from build123d import *

# Parameters (mm, degrees)
SKETCH1_W                = 369
SKETCH1_H                = 203
BOSS_EXTRUDE1_DEPTH      = 20
SKETCH2_W                = 129
SKETCH2_H                = 16
BOSS_EXTRUDE2_DEPTH      = 12
SKETCH3_W                = 342
SKETCH3_H                = 171
CUT_EXTRUDE1_DEPTH       = 9
SKETCH4_W                = 100
SKETCH4_H                = 12
BOSS_EXTRUDE3_DEPTH      = 60
CUT_EXTRUDE3_START       = -60
CUT_EXTRUDE3_DEPTH       = 70
BOSS_EXTRUDE5_DEPTH      = 40
EXTRUDE_THIN1_DEPTH      = 7
SKETCH10_W               = 404
SKETCH10_H               = 324.796202869
CUT_EXTRUDE4_DEPTH       = 69
CUT_EXTRUDE7_DEPTH       = 284.607563369
CUT_EXTRUDE7_DEPTH_BACK  = 284.607563369
SKETCH14_W               = 37
SKETCH14_H               = 34.717467541
SKETCH12_W               = 50
SKETCH12_H               = 11
BOSS_EXTRUDE6_DEPTH      = 20
SKETCH13_R               = 4
CUT_EXTRUDE6_DEPTH       = 237.312293375
CUT_EXTRUDE9_DEPTH       = 235.150592568
SKETCH16_W               = 11.814467108
SKETCH16_H               = 18.387579902
CUT_EXTRUDE10_DEPTH      = 298.007154796
BOSS_EXTRUDE8_START      = -7
SKETCH18_W               = 7.945182936
SKETCH18_H               = 20.540998505
BOSS_EXTRUDE8_DEPTH      = 7
BOSS_EXTRUDE9_START      = -7
SKETCH19_W               = 10.87781478
SKETCH19_H               = 4
BOSS_EXTRUDE9_DEPTH      = 7
FILLET1_R                = 1.5
CUT_EXTRUDE11_DEPTH      = 298.007154796
CUT_EXTRUDE11_DEPTH_BACK = 298.007154796
SKETCH20_W               = 10
SKETCH20_H               = 2.9
SKETCH21_W               = 8.352928008
SKETCH21_H               = 52
SKETCH21_W_2             = 6.5
CUT_EXTRUDE12_DEPTH      = 149.238161416
SKETCH22_W               = 43.183103185
SKETCH22_H               = 12.42943685
CUT_EXTRUDE13_DEPTH      = 298.007154796


with BuildPart() as part:
    # Sketch1 → Boss-Extrude1 (new body)
    with BuildSketch(Plane(origin=(0, 0, 0), x_dir=(1, 0, 0), z_dir=(0, 1, 0))):
        Rectangle(SKETCH1_W, SKETCH1_H)
    extrude(amount=BOSS_EXTRUDE1_DEPTH)

    # Sketch2 → Boss-Extrude2 (add)
    with BuildSketch(Plane(origin=(0, 20, 0), x_dir=(1, 0, 0), z_dir=(0, 1, 0))):
        Polygon((-184.5, -101.5), (-169.5, -101.5), (-119.5, -101.5), (-119.5, -85.5), (-169.5, -85.5), (-169.5, -36.5), (-184.5, -36.5), align=None)
        Polygon((-184.5, 101.5), (-169.5, 101.5), (-119.5, 101.5), (-119.5, 85.5), (-169.5, 85.5), (-169.5, 36.5), (-184.5, 36.5), align=None)
        with Locations((20, -93.5)):
            Rectangle(SKETCH2_W, SKETCH2_H)
        with Locations((20, 93.5)):
            Rectangle(SKETCH2_W, SKETCH2_H)
    extrude(amount=BOSS_EXTRUDE2_DEPTH)

    # Sketch3 → Cut-Extrude1 (cut)
    with BuildSketch(Plane(origin=(0, 20, 0), x_dir=(1, 0, 0), z_dir=(0, 1, 0))):
        with Locations((1.5, 0)):
            Rectangle(SKETCH3_W, SKETCH3_H)
    extrude(amount=-CUT_EXTRUDE1_DEPTH, mode=Mode.SUBTRACT)

    # Sketch4 → Boss-Extrude3 (add)
    with BuildSketch(Plane(origin=(0, 0, -101.5), x_dir=(-1, 0, 0), z_dir=(0, 0, -1))):
        with Locations((-19.5, 26)):
            Rectangle(SKETCH4_W, SKETCH4_H)
    boss_extrude3 = extrude(amount=BOSS_EXTRUDE3_DEPTH)

    # Sketch6 → Cut-Extrude3 (cut)
    with BuildSketch(Plane.XY.offset(-85.5).offset(CUT_EXTRUDE3_START)):
        with BuildLine():
            Line((-24.5, 32), (-26.787099163, 29.101539441))
            ThreePointArc((-26.787099163, 29.101539441), (-26.9948908, 27.190971116), (-25.366310671, 26.170591063))
            Line((-25.366310671, 26.170591063), (-15.633690062, 26.170591063))
            ThreePointArc((-15.633690062, 26.170591063), (-14.00510936, 27.190970786), (-14.212900837, 29.101539441))
            Line((-14.212900837, 29.101539441), (-16.5, 32))
            Line((-16.5, 32), (-24.5, 32))
        make_face()
        with BuildLine():
            Line((56.5, 32), (54.250139337, 28.697067806))
            ThreePointArc((54.250139337, 28.697067806), (54.153814675, 26.972097696), (55.633689937, 26.080599221))
            Line((55.633689937, 26.080599221), (65.366310546, 26.080599221))
            ThreePointArc((65.366310546, 26.080599221), (66.846185438, 26.972097909), (66.749860663, 28.697067806))
            Line((66.749860663, 28.697067806), (64.5, 32))
            Line((64.5, 32), (56.5, 32))
        make_face()
    cut_extrude3 = extrude(amount=CUT_EXTRUDE3_DEPTH, mode=Mode.SUBTRACT)

    # Sketch8 → Boss-Extrude5 (add)
    with BuildSketch(Plane(origin=(0, 32, 0), x_dir=(1, 0, 0), z_dir=(0, 1, 0))):
        Polygon((-184.5, 36.5), (-169.5, 36.5), (-169.5, 85.5), (-119.5, 85.5), (-119.5, 101.5), (-184.5, 101.5), align=None)
    boss_extrude5 = extrude(amount=BOSS_EXTRUDE5_DEPTH)

    # Sketch9 → Extrude-Thin1 (add)
    with BuildSketch(Plane(origin=(0, 72, 0), x_dir=(1, 0, 0), z_dir=(0, 1, 0))):
        Polygon((-119.5, 85.5), (-119.5, 71.5), (-155.5, 71.5), (-155.5, 35), (-169.5, 35), (-169.5, 45), (-165.5, 45), (-165.5, 81.5), (-129.5, 81.5), (-129.5, 85.5), align=None)
    extrude_thin1 = extrude(amount=-EXTRUDE_THIN1_DEPTH)

    # Mirror2: Boss-Extrude3, Cut-Extrude3, Boss-Extrude5, Extrude-Thin1 across plane
    add(boss_extrude3.mirror(Plane.XY))
    add(cut_extrude3.mirror(Plane.XY), mode=Mode.SUBTRACT)
    add(boss_extrude5.mirror(Plane.XY))
    add(extrude_thin1.mirror(Plane.XY))

    # Sketch10 → Cut-Extrude4 (cut)
    with BuildSketch(Plane(origin=(0, 32, 0), x_dir=(1, 0, 0), z_dir=(0, 1, 0))):
        with Locations((98.05, -0.89352463)):
            Rectangle(SKETCH10_W, SKETCH10_H)
    extrude(amount=-CUT_EXTRUDE4_DEPTH, mode=Mode.SUBTRACT)

    # Sketch14 → Cut-Extrude7 (cut, two sides: drawn at the far end of the back side and taken through both)
    with BuildSketch(Plane(origin=(0, 0, -101.5), x_dir=(-1, 0, 0), z_dir=(0, 0, -1)).offset(-CUT_EXTRUDE7_DEPTH_BACK)):
        with Locations((138, 36.253686327)):
            Rectangle(SKETCH14_W, SKETCH14_H)
    extrude(amount=CUT_EXTRUDE7_DEPTH + CUT_EXTRUDE7_DEPTH_BACK, mode=Mode.SUBTRACT)

    # Sketch12 → Boss-Extrude6 (add)
    with BuildSketch(Plane.ZY.offset(184.5)):
        with Locations((-25, 5.5)):
            Rectangle(SKETCH12_W, SKETCH12_H)
    boss_extrude6 = extrude(amount=BOSS_EXTRUDE6_DEPTH)

    # Sketch13 → Cut-Extrude6 (cut, through all)
    with BuildSketch(Plane(origin=(0, 11, 0), x_dir=(1, 0, 0), z_dir=(0, 1, 0))):
        with Locations(Location((-194.5, 25, 0), (0, 0, 270))):
            Circle(SKETCH13_R)
    cut_extrude6 = extrude(amount=-CUT_EXTRUDE6_DEPTH, mode=Mode.SUBTRACT)

    # Mirror3: Boss-Extrude6, Cut-Extrude6 across plane
    add(boss_extrude6.mirror(Plane.XY))
    add(cut_extrude6.mirror(Plane.XY), mode=Mode.SUBTRACT)

    # Sketch11 → Cut-Extrude9 (cut, through all)
    with BuildSketch(Plane(origin=(0, 20, 0), x_dir=(1, 0, 0), z_dir=(0, 1, 0))):
        Polygon((-103.95, 97.75), (-103.95, 89.25), (-111.95, 87.839384154), (-111.95, 99.160615846), align=None)
        Polygon((-103.95, -89.25), (-103.95, -97.75), (-111.95, -99.160615846), (-111.95, -87.839384154), align=None)
    extrude(amount=-CUT_EXTRUDE9_DEPTH, mode=Mode.SUBTRACT)

    # Sketch16 → Cut-Extrude10 (cut, through all)
    with BuildSketch(Plane.XY.offset(101.5)):
        with Locations((-125.407233554, 62.806210049)):
            Rectangle(SKETCH16_W, SKETCH16_H)
    extrude(amount=-CUT_EXTRUDE10_DEPTH, mode=Mode.SUBTRACT)

    # Sketch18 → Boss-Extrude8 (add)
    with BuildSketch(Plane(origin=(0, 72, 0), x_dir=(1, 0, 0), z_dir=(0, 1, 0)).offset(BOSS_EXTRUDE8_START)):
        with Locations((-135.287058576, -81.770499253)):
            Rectangle(SKETCH18_W, SKETCH18_H)
    extrude(amount=BOSS_EXTRUDE8_DEPTH)

    # Sketch19 → Boss-Extrude9 (add)
    with BuildSketch(Plane(origin=(0, 72, 0), x_dir=(1, 0, 0), z_dir=(0, 1, 0)).offset(BOSS_EXTRUDE9_START)):
        with Locations((-136.753374498, 83.5)):
            Rectangle(SKETCH19_W, SKETCH19_H)
    extrude(amount=BOSS_EXTRUDE9_DEPTH)

    # Fillet1
    fillet1_edges = [part.edges().sort_by_distance(p)[0] for p in [
        (-111.95, 10, -99.160615846),
        (-103.95, 10, -97.75),
        (-103.95, 10, -89.25),
        (-111.95, 10, -87.839384154),
        (-111.95, 10, 99.160615846),
        (-111.95, 10, 87.839384154),
        (-103.95, 10, 89.25),
        (-103.95, 10, 97.75),
    ]]
    fillet(fillet1_edges, radius=FILLET1_R)

    # Sketch20 → Cut-Extrude11 (cut, two sides: drawn at the far end of the back side and taken through both)
    with BuildSketch(Plane.XY.offset(101.5).offset(-CUT_EXTRUDE11_DEPTH_BACK)):
        with Locations((-151.5, 17.444952557)):
            Rectangle(SKETCH20_W, SKETCH20_H)
    extrude(amount=CUT_EXTRUDE11_DEPTH + CUT_EXTRUDE11_DEPTH_BACK, mode=Mode.SUBTRACT)

    # Sketch21 → Cut-Extrude12 (cut, through all)
    with BuildSketch(Plane.ZY.offset(184.5)):
        with Locations((-37.323535996, 46)):
            Rectangle(SKETCH21_W, SKETCH21_H)
        with Locations((38.25, 46)):
            Rectangle(SKETCH21_W_2, SKETCH21_H)
    extrude(amount=-CUT_EXTRUDE12_DEPTH, mode=Mode.SUBTRACT)

    # Sketch22 → Cut-Extrude13 (cut, through all)
    with BuildSketch(Plane.XY.offset(101.5)):
        with Locations((-124.908448408, 22.209670982)):
            Rectangle(SKETCH22_W, SKETCH22_H)
    extrude(amount=-CUT_EXTRUDE13_DEPTH, mode=Mode.SUBTRACT)


solid = part.part
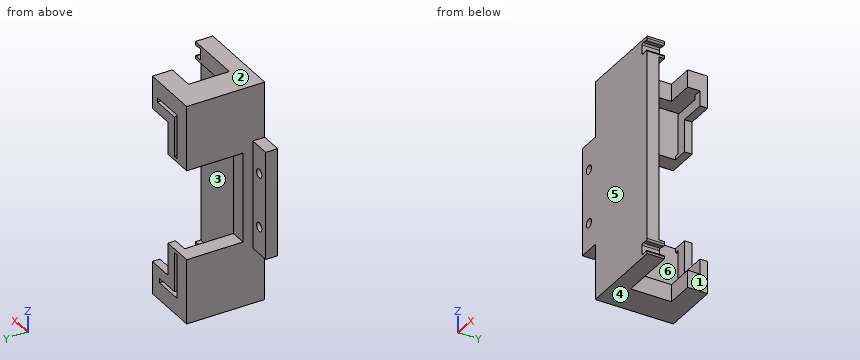
Design review of the part built by this model. Coordinates are the model's own, in mm. Face numbers are marked on the shaded views. A direction names the side the tool comes from. Coordinates: 2 decimals unless noted, no trailing zeros. Order: outer loops, then holes, each group sorted by start corner. A loop starts at its lowest first (then second) coordinate and runs counter-clockwise, first axis right, second up. Notation, with made-up numbers: (79.25, 5.5) - (123.25, 5.5) arc R9 cw to (123.25, 11.5) - close; hole circle Ø1 at (-32, 61.25). An arc over 180 degrees is marked (long way). Put each result on its own line as item: value.
1) The part is to be moulded in two halves that separate along Z. For the marked faces 3, 4, 5 and 6, say which applies: released by +Z, released by -Z, zero draft, split by the parting line, or undercut.
Response values:
face 3: undercut
face 4: released by -Z
face 5: zero draft
face 6: undercut
2) Take a section at B-B, the plane x = -194.5. Give the boundary of the cut face in (y, z).
Response values:
outline: (0, -50) - (11, -50) - (11, -29) - (0, -29) - close; (0, -21) - (11, -21) - (11, 21) - (0, 21) - close; (0, 29) - (11, 29) - (11, 50) - (0, 50) - close
3) Take a section at A-A, the plane z = -63. Give the boundary of the cut face in (x, y), and give its area (3 significant figures).
Response values:
outline: (-184.5, 0) - (-103.95, 0) - (-103.95, 11) - (-169.5, 11) - (-169.5, 72) - (-184.5, 72) - close; (-165.5, 65) - (-155.5, 65) - (-155.5, 72) - (-165.5, 72) - close
area: 1,870 mm²
4) Take a section at C-C, the plane y = 61.5. Give the boundary of the cut face in (x, z), and give its area (3 significant figures).
Response values:
outline: (-184.5, -101.5) - (-131.31, -101.5) - (-131.31, -85.5) - (-169.5, -85.5) - (-169.5, -41.5) - (-184.5, -41.5) - close; (-184.5, 41.5) - (-169.5, 41.5) - (-169.5, 85.5) - (-131.31, 85.5) - (-131.31, 101.5) - (-184.5, 101.5) - close
area: 3,020 mm²
5) Insertion check: P1, Ø5.5, axis at x = -191, y = 4.5, coming from the -Z side; P2, Ø7.5, axis at y = 67, z = -63, coming from the -X side; P3, Ø16, axis at x = -199, z = -8.5, coming from the +Y side. Each pin has a flat end and moves straight along its axis. Give the tip position at first contact, or say it passes through.
Response values:
P1: stops at z = -50
P2: stops at x = -184.5
P3: stops at y = 11
6) Take a section at D-D, the plane z = -4. Give the boundary of the cut face in (x, y).
Response values:
outline: (-204.5, 0) - (-103.95, 0) - (-103.95, 11) - (-169.5, 11) - (-169.5, 20) - (-184.5, 20) - (-184.5, 11) - (-204.5, 11) - close
7) Tool access review of the marked faces 1 and 2: name each direction out of +Z, -Z, +X, -X, +Y, -Y from which nothing blocks a thin tool from reaching the whole face with its end or side.
Response values:
face 1: +Z, -Z, +X, +Y
face 2: +Z, +X, -X, +Y, -Y
8) Wall thickness on L1, parallel to Z at x = -194, y = 4; L2, parallel to X at y = 6.75, z = -25; L3, parallel to Y at x = -158.5, z = -62: over which ranges is each line inside the solid? List them lowest first. Write a range as from..to.
Response values:
L1: z = -50..-28.97, -21.03..21.03, 28.97..50
L2: x = -204.5..-198.5, -190.5..-103.95
L3: y = 0..11, 65..72
